Read the model definition and answer for the solid it produces. Units are mm, in the model's axes. Face numbers are marked on the shaded views. Give positions to 0.01 mm unless a question says otherwise; leave off trailing zeros. Order: outer loops, then holes, each group sorted by start corner. A loop starts at its lowest first (then second) coordinate and runs counter-clockwise, first axis right, second up. Notation, with made-up numbers: M 28.25,87 L 61.25,87 A21 ccw 61.25,122 Z; hole C 1.5,-9.75 d7. An arc over 180 degrees is marked long. One line per item, written item: value.
from build123d import *

# Parameters (mm, degrees)
F0_W     = 94
F0_H     = 88
F0_R     = 2.5
F1_DEPTH = 10
F2_W     = 92
F2_H     = 86
F3_DEPTH = 8
F4_W     = 78.2
F4_H     = 50.94
F5_DEPTH = 25
F0_R_2   = 1.5
F6_DEPTH = 10


with BuildPart() as f1:
    # F0 (on Top) → F1 (new body)
    with BuildSketch(Plane.XY):
        with Locations((6.636954, 8.70822)):
            Rectangle(F0_W, F0_H)
        with Locations((-37.816051, -32.62452)):
            Circle(F0_R, mode=Mode.SUBTRACT)
        with Locations((51.075991, -32.724809)):
            Circle(F0_R, mode=Mode.SUBTRACT)
        with Locations((-37.748028, 50.113171)):
            Circle(F0_R, mode=Mode.SUBTRACT)
        with Locations((51.075991, 50.113171)):
            Circle(F0_R, mode=Mode.SUBTRACT)
    extrude(amount=F1_DEPTH)

    # F2 (on Top) → F3 (cut)
    with BuildSketch(Plane.XY):
        with Locations((6.636954, 8.70822)):
            Rectangle(F2_W, F2_H)
    extrude(amount=F3_DEPTH, mode=Mode.SUBTRACT)

    # F4 (on Top) → F5 (cut)
    with BuildSketch(Plane.XY):
        with Locations((6.036954, 17.67822)):
            Rectangle(F4_W, F4_H)
    extrude(amount=F5_DEPTH, mode=Mode.SUBTRACT)

    # F0 (on Top) → F6 (join)
    with BuildSketch(Plane.XY):
        with Locations((-37.816051, -32.62452)):
            Circle(F0_R)
        with Locations((-37.816051, -32.62452)):
            Circle(F0_R_2, mode=Mode.SUBTRACT)
        with Locations((-37.748028, 50.113171)):
            Circle(F0_R)
        with Locations((-37.748028, 50.113171)):
            Circle(F0_R_2, mode=Mode.SUBTRACT)
        with Locations((51.075991, 50.113171)):
            Circle(F0_R)
        with Locations((51.075991, 50.113171)):
            Circle(F0_R_2, mode=Mode.SUBTRACT)
        with Locations((51.075991, -32.724809)):
            Circle(F0_R)
        with Locations((51.075991, -32.724809)):
            Circle(F0_R_2, mode=Mode.SUBTRACT)
    extrude(amount=F6_DEPTH)


solid = f1.part
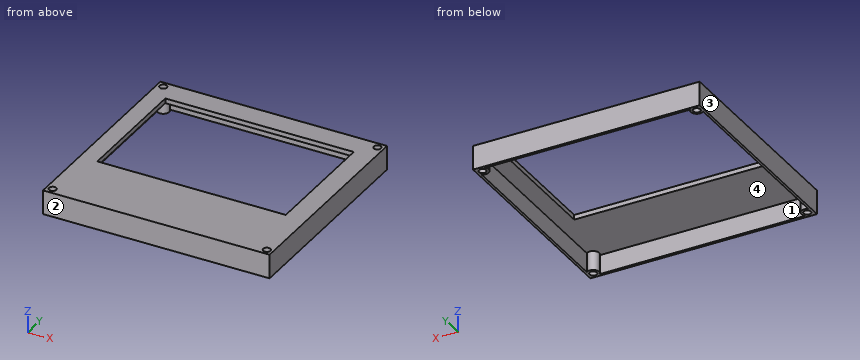
1) Find section C-C, the plane z = 3.5. Write down the section's boundary in (x, y), plus the area to 3 significant figures.
Reported:
outline: M -40.36,-35.29 L 53.64,-35.29 L 53.64,52.71 L -40.36,52.71 Z; hole M -39.36,-30.66 A2.5 cw -35.95,-34.29 L 49.13,-34.29 A2.5 cw 52.64,-30.77 L 52.64,48.16 A2.5 cw 49.15,51.71 L -35.82,51.71 A2.5 cw -39.36,48.2 Z; hole C -37.82,-32.62 d3; hole C -37.75,50.11 d3; hole C 51.08,-32.72 d3; hole C 51.08,50.11 d3
area: 391 mm^2
2) This flat-tipped pin is pushed along its axis until it touches: pin 1 Ø1.5 at (x, y) = (39.5, -22) entering from -Z. Where does it stop, or does it pass through?
Reported:
pin 1: stops at z = 8
3) Determine the mould class of the marked faces 1, 2, 3 and 4 for opening direction X: +X half, -X half, draft (parallel to the pull), parting line (faces both ways), or undercut.
Reported:
face 1: undercut
face 2: draft
face 3: -X half
face 4: undercut
4) Consider probe 1 along Y at (x, z) = (28, 3); probe 2 along X at (y, z) = (10, 6); probe 3 along Y at (x, z) = (-13.5, 9.75). Determine where each line is inside the solid, lowest interval first.
Reported:
probe 1: y = -35.29 to -34.29, 51.71 to 52.71
probe 2: x = -40.36 to -39.36, 52.64 to 53.64
probe 3: y = -35.29 to -7.79, 43.15 to 52.71
5) Find section D-D, the plane x = 47.5. Write down the section's boundary in (y, z), plus the area to 3 significant figures.
Reported:
outline: M -35.29,0 L -34.29,0 L -34.29,8 L 51.71,8 L 51.71,0 L 52.71,0 L 52.71,10 L -35.29,10 Z
area: 192 mm^2
6) Find section B-B, the plane x = -21.5. Write down the section's boundary in (y, z).
Reported:
outline: M -35.29,0 L -34.29,0 L -34.29,8 L -7.79,8 L -7.79,10 L -35.29,10 Z; M 43.15,8 L 51.71,8 L 51.71,0 L 52.71,0 L 52.71,10 L 43.15,10 Z
7) Find section A-A, the plane y = 25. Write down the section's boundary in (x, z).
Reported:
outline: M -40.36,0 L -39.36,0 L -39.36,8 L -33.06,8 L -33.06,10 L -40.36,10 Z; M 45.14,8 L 52.64,8 L 52.64,0 L 53.64,0 L 53.64,10 L 45.14,10 Z
